The drawing under review shows one solid part. Ordinate dimensions are in mm from its lowest x, y, z. Round coordinates to 2 decimals unless told otherwise and drop trailing zeros. Write each loop counter-clockwise with the first axis right and the second up, starting at its lowest first coordinate (ties: lowest second). Pieces come first, ordered by that corner, then holes. Notation, with made-up numbers: (72, 44) -> (113, 44) arc R34 cw to (113, 74) -> close; hole circle Ø9 at (69.5, 4.5). An arc over 180 degrees is marked (long way). Use CSV: the item, a comma, the result in double quotes. Start each with the question number.
1) Take a section at A-A, the plane z = 255. Give the boundary of the cut face in (x, y).
2) Wall thickness on probe 1 along X at (y, z) = (1.85, 150); probe 2 along Z at (x, y) = (26.5, 0.85); probe 3 along Z at (x, y) = (5.5, 2.2): over which ranges is each line inside the solid? List them lowest first. Write a range as [from, to].
3) Take a section at B-B, the plane y = 2.8. State how many separate pieces and enclosed holes the cut face has, then the cut area to 3 significant figures.
4) For pin 1 Ø3 at (x, z) = (100, 255) entering from -Y, flat-tipped, find the tip position at first contact; note if it passes through.
5) Take a section at D-D, the plane z = 10. Give the boundary of the cut face in (x, y).
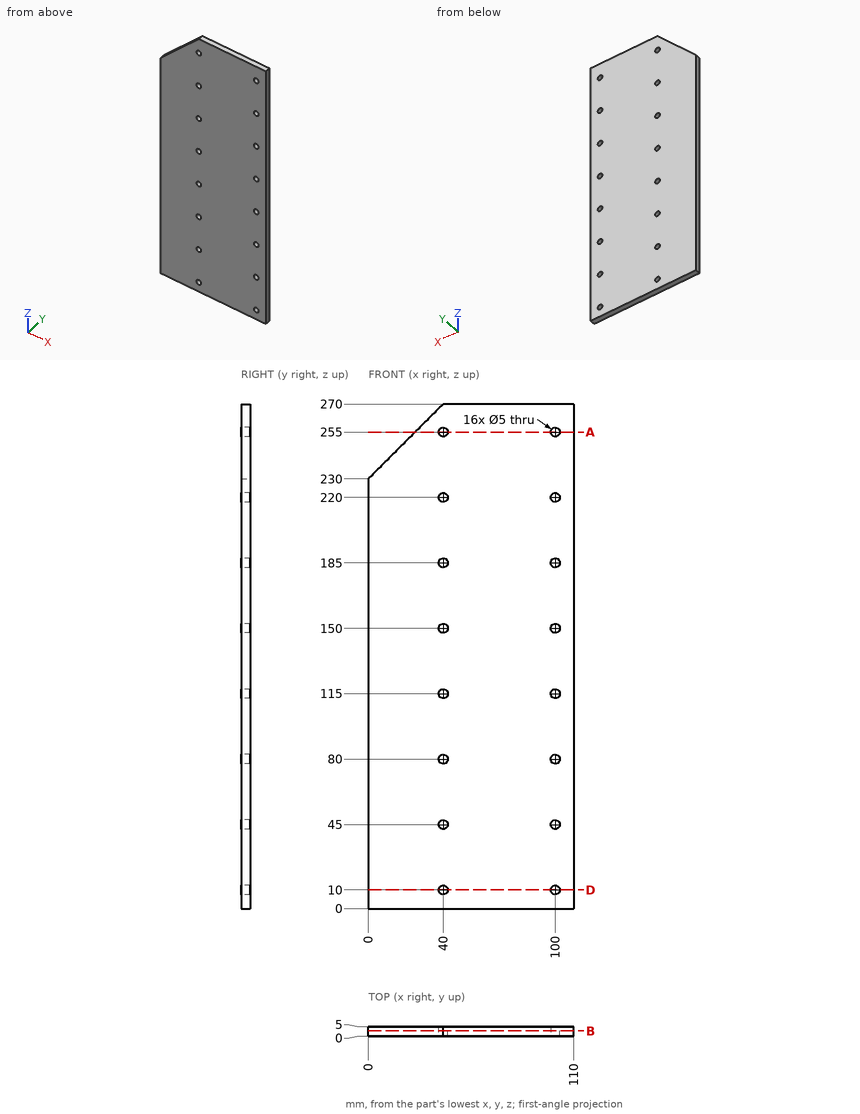
Values found:
1,outline,"(25, 0) -> (37.5, 0) -> (37.5, 5) -> (25, 5) -> close; (42.5, 0) -> (97.5, 0) -> (97.5, 5) -> (42.5, 5) -> close; (102.5, 0) -> (110, 0) -> (110, 5) -> (102.5, 5) -> close"
2,probe 1,"[0, 37.5], [42.5, 97.5], [102.5, 110]"
2,probe 2,"[0, 256.5]"
2,probe 3,"[0, 235.5]"
3,separate pieces,"1"
3,enclosed holes,"16"
3,area,"28,600 mm²"
4,pin 1,"through"
5,outline,"(0, 0) -> (37.5, 0) -> (37.5, 5) -> (0, 5) -> close; (42.5, 0) -> (97.5, 0) -> (97.5, 5) -> (42.5, 5) -> close; (102.5, 0) -> (110, 0) -> (110, 5) -> (102.5, 5) -> close"
